Here's how the part is built. I have some questions about the finished solid (model axes, mm). Face numbers are marked on the shaded views. A direction names the side the tool comes from. Give positions to 0.01 mm unless a question says otherwise; leave off trailing zeros. Loops run counter-clockwise (first coordinate to the right, second up) from the corner with the lowest first, then second, coordinate; pieces in that order, holes last. Notation, with made-up numbers: (58.25, 41.5) - (84.25, 41.5) arc R10 cw to (84.25, 53.5) - close; hole circle Ø6 at (74.5, -4). An arc over 180 degrees is marked (long way). Use one line per item in the form item = value.
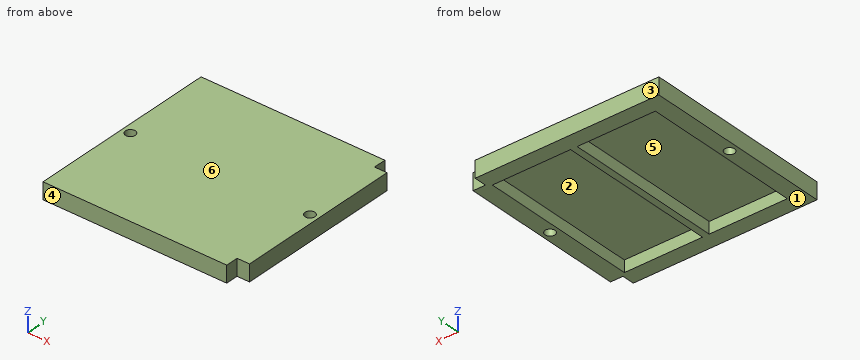
from build123d import *

# Parameters (mm, degrees)
F0_W     = 118
F0_H     = 115
F0_R     = 3
F2_DEPTH = 10
F1_W     = 47
F1_H     = 96
F3_DEPTH = 7
F4_W     = 7.5
F4_H     = 7.5
F5_DEPTH = 25


with BuildPart() as f2:
    # F0 (on Top) → F2 (new body)
    with BuildSketch(Plane.XY):
        Rectangle(F0_W, F0_H)
        with Locations((-54, 0)):
            Circle(F0_R, mode=Mode.SUBTRACT)
        with Locations((54, 0)):
            Circle(F0_R, mode=Mode.SUBTRACT)
    extrude(amount=F2_DEPTH)

    # F1 (on Top) → F3 (cut)
    with BuildSketch(Plane.XY):
        with Locations((-25.5, 0)):
            Rectangle(F1_W, F1_H)
        with Locations((25.5, 0)):
            Rectangle(F1_W, F1_H)
    extrude(amount=F3_DEPTH, mode=Mode.SUBTRACT)

    # F4 (on Top) → F5 (cut)
    with BuildSketch(Plane.XY):
        with Locations((55.25, -53.75)):
            Rectangle(F4_W, F4_H)
        with Locations((55.25, 53.75)):
            Rectangle(F4_W, F4_H)
    extrude(amount=F5_DEPTH, mode=Mode.SUBTRACT)


solid = f2.part
(1) Thinking about a two-plate mould opening in Y: for the marked faces 3, 4, 5 and 6, which applies, pulls with the +Y half, pulls with the -Y half, needs draft (parallel to the pull), parting line crosses it, or undercut?
Geometry says:
face_3 = pulls with the +Y half
face_4 = pulls with the -Y half
face_5 = undercut
face_6 = needs draft
(2) If we section it at B-B (x = -54): List the corners of the cut face in (y, z) for me.
Geometry says:
outline = (-57.5, 0) - (-3, 0) - (-3, 10) - (-57.5, 10) - close; (3, 0) - (57.5, 0) - (57.5, 10) - (3, 10) - close
(3) For P1, Ø23.5, axis at x = -16.5, y = -2, coming from the -Z side; P2, Ø6, axis at x = 55, z = 3.5, coming from the -Y side; P3, Ø2, axis at x = 56, z = 5.5, coming from the +Y side, each with a flat end and sliding along its axis, tell me the tip position at first contact or that it passes through.
Geometry says:
P1 = 7
P2 = -50
P3 = 50
(4) If we section it at D-D (x = -41): List the corners of the cut face in (y, z) for me, plus the area to 3 significant figures.
Geometry says:
outline = (-57.5, 0) - (-48, 0) - (-48, 7) - (48, 7) - (48, 0) - (57.5, 0) - (57.5, 10) - (-57.5, 10) - close
area = 478 mm²
(5) If we section it at A-A (y = 0): List the corners of the cut face in (x, z) for me, plus the area to 3 significant figures.
Geometry says:
outline = (-59, 0) - (-57, 0) - (-57, 10) - (-59, 10) - close; (-51, 0) - (-49, 0) - (-49, 7) - (-2, 7) - (-2, 0) - (2, 0) - (2, 7) - (49, 7) - (49, 0) - (51, 0) - (51, 10) - (-51, 10) - close; (57, 0) - (59, 0) - (59, 10) - (57, 10) - close
area = 402 mm²
(6) For the marked faces 1 and 2, which set-ups out of +Z, -Z, +X, -X, +Y, -Y let a thin tool reach every point of the face, with its end or its side?
Geometry says:
face_1 = -Z, +X, -X, +Y, -Y
face_2 = -Z
(7) If I drill on probe 1 along X at (y, z) = (-28, 1); probe 2 along Y at (x, z) = (-14.5, 2); probe 3 along X at (y, z) = (-2.5, 6.5), over which ranges is the centre line in solid material (lowest first)?
Geometry says:
probe_1 = -59 to -49, -2 to 2, 49 to 59
probe_2 = -57.5 to -48, 48 to 57.5
probe_3 = -59 to -55.66, -52.34 to -49, -2 to 2, 49 to 52.34, 55.66 to 59
(8) If we section it at C-C (y = 24): List the corners of the cut face in (x, z) for me.
Geometry says:
outline = (-59, 0) - (-49, 0) - (-49, 7) - (-2, 7) - (-2, 0) - (2, 0) - (2, 7) - (49, 7) - (49, 0) - (59, 0) - (59, 10) - (-59, 10) - close
